```python
from build123d import *

# Parameters (mm, degrees)
F0_R         = 15
F1_DEPTH     = 100
F1_FACE_R    = 15
F3_R         = 12
F6_R         = 8
F4_FACE_R    = 12
F8_DEPTH     = 8
F8_FACE_R    = 8
F10_R        = 5.25
F12_DEPTH    = 28
F13_T        = 0.2
F13_T4_ANGLE = 180.000000001
F13_T6_ANGLE = 180.000000001


# Not quite as in the source:
# - a shell that OpenCascade refuses in one call is made with other operations: the cavity is built on its own and cut out


with BuildPart() as f1:
    # F0 (on Front) → F1 (new body)
    with BuildSketch(Plane.XZ):
        Circle(F0_R)
    extrude(amount=-F1_DEPTH)

    # F1_face (on face) → F4 section 0
    with BuildSketch(Plane(origin=(0, 100, 0), x_dir=(1, 0, 0), z_dir=(0, 1, 0))):
        Circle(F1_FACE_R)
    # F3 (on offset) → F4 section 1
    with BuildSketch(Plane(origin=(0, 105, 0), x_dir=(-1, 0, 0), z_dir=(0, 1, 0))):
        Circle(F3_R)
    loft()

    # F6 (on offset) → F7 section 0
    with BuildSketch(Plane(origin=(0, 132, 0), x_dir=(-1, 0, 0), z_dir=(0, 1, 0))):
        Circle(F6_R)
    # F4_face (on face) → F7 section 1
    with BuildSketch(Plane(origin=(0, 105, 0), x_dir=(-1, 0, 0), z_dir=(0, 1, 0))):
        Circle(F4_FACE_R)
    loft()

    # F8 (add): a face of the model
    f8_faces = [f1.faces().sort_by_distance(p)[0] for p in [
        (0, 132, 0),
    ]]
    extrude(f8_faces, amount=F8_DEPTH)

    # F8_face (on face) → F11 section 0
    with BuildSketch(Plane(origin=(0, 140, 0), x_dir=(-1, 0, 0), z_dir=(0, 1, 0))):
        Circle(F8_FACE_R)
    # F10 (on offset) → F11 section 1
    with BuildSketch(Plane(origin=(0, 146.5, 0), x_dir=(-1, 0, 0), z_dir=(0, 1, 0))):
        Circle(F10_R)
    loft()

    # F12 (add): a face of the model
    f12_faces = [f1.faces().sort_by_distance(p)[0] for p in [
        (0, 146.5, 0),
    ]]
    extrude(f12_faces, amount=F12_DEPTH)

    # F13: shell of thickness 0.2, made by hand


with BuildPart() as f13_core1:
    # F13_t2: copy of F1
    add(f1.part)

    # the walls: a layer under each face that stays
    f13_faces = [f13_core1.faces().sort_by_distance(p)[0] for p in [
        (-15, 50, 0),
        (-13.5, 102.5, 0),
        (10, 118.5, 0),
        (8, 136, 0),
        (6.625, 143.25, 0),
        (5.25, 160.5, 0),
    ]]
    thicken(f13_faces, amount=-F13_T, mode=Mode.SUBTRACT)

    # F13_s3 → F13_t4 (revolve, cut)
    with BuildSketch(Plane.XY):
        Polygon((-12.0036933928, 105.0013220888), (-11.8285014149, 104.8971008489), (-11.807999158, 104.931271277), (-11.8021593075, 104.9706902678), align=None)
    revolve(axis=Axis((0, 105, 0), (0, -1, 0)), revolution_arc=F13_T4_ANGLE, mode=Mode.SUBTRACT)

    # F13_s5 → F13_t6 (revolve, cut)
    with BuildSketch(Plane.XY):
        Polygon((12.0036933928, 105.0013220888), (11.8285014149, 104.8971008489), (11.807999158, 104.931271277), (11.8021593075, 104.9706902678), align=None)
    revolve(axis=Axis((0, 105, 0), (0, -1, 0)), revolution_arc=F13_T6_ANGLE, mode=Mode.SUBTRACT)

    # F13_s7 → F13_t8 (revolve, cut)
    with BuildSketch(Plane.XY):
        Polygon((-8.0039784069, 132.0002930973), (-7.8021593075, 131.9706902678), (-7.8, 131.9852655936), (-7.8, 132), align=None)
    revolve(axis=Axis((0, 132, 0), (0, 1, 0)), mode=Mode.SUBTRACT)

    # F13_s9 → F13_t10 (revolve, cut)
    with BuildSketch(Plane.XY):
        Polygon((-5.2538419345, 146.50077928), (-5.0658065498, 146.4220720018), (-5.05, 146.4594329377), (-5.05, 146.5), align=None)
    revolve(axis=Axis((0, 146.5, 0), (0, 1, 0)), mode=Mode.SUBTRACT)


with BuildPart() as f1_1:
    add(f1.part)

    # what is left inside the walls is the cavity
    f13_cavity = [f13_core1.part.solids().sort_by_distance(p)[0] for p in [
        (-14.798, 66.629735, 0),
    ]]
    add(f13_cavity, mode=Mode.SUBTRACT)


solid = f1_1.part
```
The listing builds one solid part. Answer for the finished solid, in the listing's coordinates (mm). A direction names the side the tool comes from. Give positions to 0.01 mm unless a question says otherwise; leave off trailing zeros. Write each loop counter-clockwise with the first axis right and the second up, starting at its lowest first coordinate (ties: lowest second). Pieces come first, ordered by that corner, then holes. Notation, with made-up numbers: (18, 26) -> (57, 26) arc R9 ccw to (57, 35) -> close; hole circle Ø9 at (-37.5, 25). An arc over 180 degrees is marked (long way). Write item = value, one per line. Start each with the question number.
1) The part is cut by section B-B, the plane y = 126. Determine the outline of the cut face in (x, z).
2) Which of the six approach directions +Z, -Z, +X, -X, +Y, -Y give full straight-line access (tool end or side, diameter ignored) to faces 3 (the face through (5.75, 135.92, 5.27)), 4 (the face through (-14.985, 49.3, 0.66)), 5 (the face through (-5, 160.3, 1.6))?
3) Determine the mould class of faces 1 (the face through (-9.263, 118.311, -3.841)), 2 (the face through (-4.817, 160.283, 1.517)) for opening direction Z: +Z half, -Z half, draft (parallel to the pull), parting line (faces both ways), or undercut.
4) The part is cut by section A-A, the plane y = 63.5. Determine the outline of the cut face in (x, z), and give its area (3 significant figures).
5) Each of these flat-tipped pins is pushed along its axis until it touches: pin 1 (1 mm diameter, centred on x = 5.5, y = 97, fed in from +Z); pin 2 (5 mm diameter, centred on x = 4.5, y = 142, fed in from +Z); pin 3 (2 mm diameter, centred on x = -11.5, z = 6, fed in from -Y); pin 4 (12.5 mm diameter, centred on x = 0, z = 0, fed in from +Y). Where does it stop, or does it pass through?
6) Straight lines are drawn through the part: line 1 along Z through (x, y) = (0, 155); line 2 along Z through (x, y) = (0, 59); line 3 along X through (y, z) = (129.5, 2). For each, find the intervals that lie inside material, in ascending order.
Solutions:
q1.outline = circle Ø17.78 at (0, 0); hole circle Ø17.37 at (0, 0)
q2.face_3 = -Y
q2.face_4 = +Y, -Y
q2.face_5 = +Y
q3.face_1 = parting line
q3.face_2 = undercut
q4.outline = circle Ø30 at (0, 0); hole circle Ø29.6 at (0, 0)
q4.area = 18.7 mm²
q5.pin_1 = 14.14
q5.pin_2 = 7.42
q5.pin_3 = 101.33
q5.pin_4 = 174.5
q6.line_1 = -5.25 to -5.05, 5.05 to 5.25
q6.line_2 = -15 to -14.8, 14.8 to 15
q6.line_3 = -8.13 to -7.92, 7.92 to 8.13
